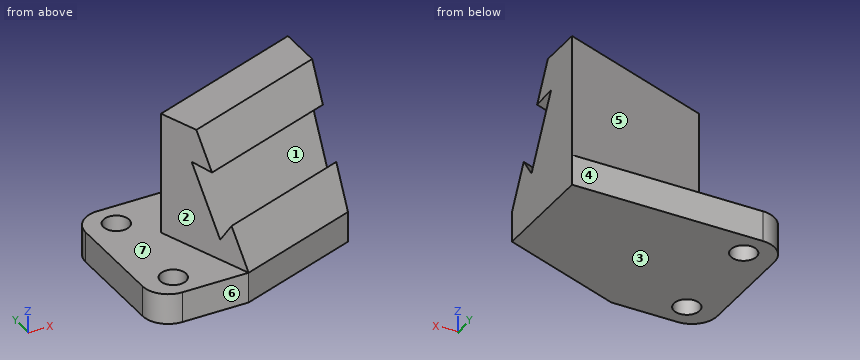
from build123d import *

# Parameters (mm, degrees)
F0_R     = 6.3
F1_DEPTH = 15
F2_DEPTH = 75
F4_DEPTH = 83.0489551508


with BuildPart() as f1:
    # F0 (on Top) → F1 (new body)
    with BuildSketch(Plane.XY):
        with BuildLine():
            Line((0, 62.5), (0, 12.5))
            ThreePointArc((0, 12.5), (3.6611652352, 3.6611652352), (12.5, 0))
            Line((12.5, 0), (45, 0))
            Line((45, 0), (28.0404697245, 46.5959264764))
            Line((28.0404697245, 46.5959264764), (106.0800203511, 75))
            Line((106.0800203511, 75), (12.5, 75))
            ThreePointArc((12.5, 75), (3.6611652352, 71.3388347648), (0, 62.5))
        make_face()
        with Locations((15, 12.5)):
            Circle(F0_R, mode=Mode.SUBTRACT)
        with Locations((15, 62.5)):
            Circle(F0_R, mode=Mode.SUBTRACT)
    extrude(amount=F1_DEPTH)

    # F0 (on Top) → F2 (join)
    with BuildSketch(Plane.XY):
        Polygon((28.0404697245, 46.5959264764), (45, 0), (106.0800203511, 22.2313093162), (106.0800203511, 75), align=None)
    extrude(amount=F2_DEPTH)

    # F3 (on face) → F4 (cut, through all)
    with BuildSketch(Plane(origin=(39.7359999702, 14.4627212179, 0), x_dir=(0.3420201433, -0.9396926208, 0), z_dir=(-0.9396926208, -0.3420201433, 0))):
        Polygon((-0.7092158589, 25.0393128685), (5.70626248, 34.6400925773), (-5.3502404503, 57.0622633677), (-16.8724987437, 57.8178407322), align=None)
        Polygon((5.70626248, 34.6400925773), (15.3909064497, 15), (15.3909064497, 75), (-14.1954427945, 75), (-5.3502404503, 57.0622633677), align=None)
    extrude(amount=-F4_DEPTH, mode=Mode.SUBTRACT)


solid = f1.part
Part model, mm, in its own coordinate system. Face numbers are marked on the shaded views. A direction names the side the tool comes from. Give positions to 0.01 mm unless a question says otherwise; leave off trailing zeros. Write each loop counter-clockwise with the first axis right and the second up, starting at its lowest first coordinate (ties: lowest second). Pieces come first, ordered by that corner, then holes.
1) Cut at D-D on x = 26.5. Write the cut outline in (y, z), then the cut area to 4 significant figures.
Resolved:
outline: (0, 0) - (75, 0) - (75, 15) - (0, 15) - close
area: 1,125 mm2
2) Probe L1, parallel to Y at x = 15, z = 8.75; L2, parallel to X at y = 62, z = 10; L3, parallel to Z at x = 82, y = 71.5. List the from-to ranges inside material, lowest first.
Resolved:
L1: y = 0 to 6.2, 18.8 to 56.2, 68.8 to 75
L2: x = 0 to 8.72, 21.28 to 106.08
L3: z = 0 to 15
3) Cut at A-A on x = 15. Write the cut outline in (y, z), then the cut area to 3 significant figures.
Resolved:
outline: (0, 0) - (6.2, 0) - (6.2, 15) - (0, 15) - close; (18.8, 0) - (56.2, 0) - (56.2, 15) - (18.8, 15) - close; (68.8, 0) - (75, 0) - (75, 15) - (68.8, 15) - close
area: 747 mm2
4) Which spindle directions (+Z, -Z, +X, -X, +Y, -Y) get a long thin tool onto all of the face, cutting with end or side? Do the marked faces 5, 6 and 7. Say none if no direction does.
Resolved:
face 5: +Z, -X, +Y
face 6: +Z, -Z, +X, -X, -Y
face 7: +Z, -X
5) Cut at C-C on y = 42. Write the cut outline in (x, z), then the cut area to 3 significant figures.
Resolved:
outline: (0, 0) - (106.08, 0) - (106.08, 30.06) - (66.06, 57.82) - (99.75, 57.06) - (73.89, 75) - (29.71, 75) - (29.71, 15) - (0, 15) - close
area: 5,290 mm2
6) Cut at B-B on z = 29. Write the cut outline in (x, y), then the cut area to 3 significant figures.
Resolved:
outline: (28.04, 46.6) - (38.83, 16.96) - (106.08, 41.44) - (106.08, 75) - close; (40.4, 12.64) - (42.64, 6.49) - (106.08, 29.58) - (106.08, 36.55) - close
area: 2,890 mm2
7) Two-plate mould, pull along Y, no slides. Class the marked faces 1, 2, 3 and 4: released by +Y, released by -Y, zero draft, split by the parting line, or undercut.
Resolved:
face 1: undercut
face 2: released by -Y
face 3: zero draft
face 4: released by +Y
8) Pin check, flat tips, straight feed: pin 1 (8 mm diameter, centred on x = 74, z = 16, fed in from -Y); pin 2 (10 mm diameter, centred on x = 84.5, y = 40, fed in from +Z); pin 3 (6 mm diameter, centred on x = 55, y = 45, fed in from -Z); pin 4 (6 mm diameter, centred on y = 32, z = 41.5, fed in from -X). Stop position of each tip, or through.
Resolved:
pin 1: stops at y = 9.15
pin 2: stops at z = 73.97
pin 3: stops at z = 0
pin 4: stops at x = 32.26
